Design review of the part built by this model. Coordinates are the model's own, in mm. A direction names the side the tool comes from. Give positions to 0.01 mm unless a question says otherwise; leave off trailing zeros.
```python
from build123d import *

# Parameters (mm, degrees)
SKETCH2_R           = 3.175
SKETCH2_R_2         = 5.08
BOSS_EXTRUDE1_DEPTH = 19.05
CUT_EXTRUDE2_START  = -12.7
CUT_EXTRUDE2_DEPTH  = 6.35
CUT_EXTRUDE3_DEPTH  = 6.35


with BuildPart() as part:
    # Sketch2 → Boss-Extrude1 (new body)
    with BuildSketch(Plane(origin=(0, 0, 0), x_dir=(0, 0, -1), z_dir=(1, 0, 0))):
        with BuildLine():
            Line((270.378794472, 38.1), (21.997045256, 38.1))
            Line((21.997045256, 38.1), (-270.378794472, 38.1))
            ThreePointArc((-270.378794472, 38.1), (-273.05, 0), (-270.378794472, -38.1))
            Line((-270.378794472, -38.1), (270.378794472, -38.1))
            ThreePointArc((270.378794472, -38.1), (273.05, 0), (270.378794472, 38.1))
        make_face()
        with Locations(Location((-261.240141142, -19.100852393, 0), (0, 0, 180))):
            Circle(SKETCH2_R, mode=Mode.SUBTRACT)
        with Locations(Location((-238.949490115, -19.110830171, 0), (0, 0, 180))):
            Circle(SKETCH2_R, mode=Mode.SUBTRACT)
        with BuildLine():
            ThreePointArc((11.1125, 19.247414599), (12.274630657, 14.910283942), (7.9375, 13.748153285))
            ThreePointArc((7.9375, 13.748153285), (6.775369343, 18.085283942), (11.1125, 19.247414599))
        make_face(mode=Mode.SUBTRACT)
        with Locations(Location((-16.497783942, 9.525, 0), (0, 0, 180))):
            Circle(SKETCH2_R, mode=Mode.SUBTRACT)
        with Locations(Location((-9.525, -16.497783942, 0), (0, 0, 180))):
            Circle(SKETCH2_R, mode=Mode.SUBTRACT)
        with Locations(Location((16.497783942, -9.525, 0), (0, 0, 180))):
            Circle(SKETCH2_R, mode=Mode.SUBTRACT)
        with Locations(Location((238.949490115, -19.110830171, 0), (0, 0, 180))):
            Circle(SKETCH2_R, mode=Mode.SUBTRACT)
        with Locations(Location((261.240141142, -19.100852393, 0), (0, 0, 180))):
            Circle(SKETCH2_R, mode=Mode.SUBTRACT)
        with Locations(Location((259.820783483, 0, 0), (0, 0, 180))):
            Circle(SKETCH2_R_2, mode=Mode.SUBTRACT)
        with Locations(Location((-228.070127818, 0, 0), (0, 0, 180))):
            Circle(SKETCH2_R_2, mode=Mode.SUBTRACT)
        with Locations(Location((-164.570319717, 0, 0), (0, 0, 180))):
            Circle(SKETCH2_R_2, mode=Mode.SUBTRACT)
        with Locations(Location((-101.070508964, 0, 0), (0, 0, 180))):
            Circle(SKETCH2_R_2, mode=Mode.SUBTRACT)
        with Locations(Location((-261.240141142, 19.100852393, 0), (0, 0, 180))):
            Circle(SKETCH2_R, mode=Mode.SUBTRACT)
        with Locations(Location((-238.949490115, 19.110830171, 0), (0, 0, 180))):
            Circle(SKETCH2_R, mode=Mode.SUBTRACT)
        with Locations(Location((69.320600315, 0, 0), (0, 0, 180))):
            Circle(SKETCH2_R_2, mode=Mode.SUBTRACT)
        with Locations(Location((132.82041491, 0, 0), (0, 0, 180))):
            Circle(SKETCH2_R_2, mode=Mode.SUBTRACT)
        with Locations(Location((196.320223938, 0, 0), (0, 0, 180))):
            Circle(SKETCH2_R_2, mode=Mode.SUBTRACT)
        with Locations(Location((238.949490115, 19.110830171, 0), (0, 0, 180))):
            Circle(SKETCH2_R, mode=Mode.SUBTRACT)
        with Locations(Location((261.240141142, 19.100852393, 0), (0, 0, 180))):
            Circle(SKETCH2_R, mode=Mode.SUBTRACT)
    extrude(amount=BOSS_EXTRUDE1_DEPTH)

    # Sketch3 → Cut-Extrude2 (cut)
    with BuildSketch(Plane(origin=(19.05, 0, 0), x_dir=(0, 0, -1), z_dir=(1, 0, 0)).offset(CUT_EXTRUDE2_START)):
        Polygon((65.991135768, -38.1), (21.997045256, 38.1), (-65.991135768, 38.1), (-21.997045256, -38.1), align=None)
    extrude(amount=-CUT_EXTRUDE2_DEPTH, mode=Mode.SUBTRACT)

    # Sketch3_5 → Cut-Extrude3 (cut)
    with BuildSketch(Plane(origin=(19.05, 0, 0), x_dir=(0, 0, -1), z_dir=(1, 0, 0))):
        Polygon((21.997045256, -38.1), (65.991135768, 38.1), (-21.997045256, 38.1), (-65.991135768, -38.1), align=None)
    extrude(amount=-CUT_EXTRUDE3_DEPTH, mode=Mode.SUBTRACT)


solid = part.part
```
(1) Tool access review of faces 1 (the face through (15.92, -0.53, -43.69)), 2 (the face through (15.92, 0.53, 43.69)), 3 (the face through (3.22, -0.53, -44.3)), 4 (the face through (12.7, 1, 1)): name each direction out of +Z, -Z, +X, -X, +Y, -Y from which nothing blocks a thin tool from reaching the whole face with its end or side.
Resolved:
face 1: +X, +Y
face 2: +X, -Y
face 3: -X, -Y
face 4: +X
(2) Consider section A-A, the plane y = 0. Give the number of separate pieces and of enclosed holes in the cut face, then the cut area to 3 significant figures.
Resolved:
separate pieces: 8
enclosed holes: 0
area: 7,930 mm2
(3) Clearance check with flat-ended pins moving along their axes: P1, Ø3, axis at x = 3, z = -35.5, coming from the -Y side; P2, Ø7.5, axis at y = 9.52, z = 16.5, coming from the +X side; P3, Ø5, axis at x = 16, z = -38, coming from the +Y side. State where each tip first meets the part, or that it passes through.
Resolved:
P1: stops at y = 12.11
P2: stops at x = 12.7
P3: stops at y = -6.05
(4) To check wall thickness, follow L1, parallel to Z at x = 1.75, y = 18.5; L2, parallel to Y at x = 4, z = 228; L3, parallel to Z at x = 3, y = 30. State the ranges of each line that lie inside material, in increasing order.
Resolved:
L1: z = -272.42 to -264.36, -258.12 to -242.07, -235.83 to -33.31, 54.68 to 235.83, 242.07 to 258.12, 264.36 to 272.42
L2: y = -38.1 to -5.08, 5.08 to 38.1
L3: z = -271.4 to -26.67, 61.31 to 271.4
